Here's how the part is built. I have some questions about the finished solid (model axes, mm). Coordinates: 2 decimals unless noted, no trailing zeros. Write each loop counter-clockwise with the first axis right and the second up, starting at its lowest first coordinate (ties: lowest second). Pieces come first, ordered by that corner, then holes. Notation, with made-up numbers: M 23.5,-13.75 L 55.5,-13.75 A34 cw 55.5,25.25 Z; hole C 14.5,54 d2. An arc over 180 degrees is marked long. Use one line per item in the form item = value. Start each with the question number.
1. I want a section at D-D, the plane z = -30.5. List the corners of the cut face in (x, y) for me.
2. I want a section at C-C, the plane y = -15.5. List the corners of the cut face in (x, z) for me, plus the area to 3 significant figures.
3. I want a section at B-B, the plane x = -67. List the corners of the cut face in (y, z) for me.
4. I'm going to push flat-ended pins straight in: pin 1 Ø12 at (y, z) = (-9.5, -9) entering from +X; pin 2 Ø1 at (x, y) = (28, -15) entering from -Z; pin 3 Ø10 at (y, z) = (-9, -26.5) entering from +X. Where does each tip first touch, or does it pass through?
5. Thinking about a two-plate mould opening in Z: for faces 1 (the face through (47.98, -9.86, 35.17)), 2 (the face through (0, -10, -50)), 3 (the face through (84.87, -9.86, -1.99)), which applies, released by +Z, released by -Z, zero draft, split by the parting line, or undercut?
6. Please list where these lines run through material, in increasing order: line 1 along X through (y, z) = (-7.25, -2); line 2 along X through (y, z) = (-9.5, 12); line 3 along Z through (x, y) = (2, -13.75). Write a range as [from, to].
7. I want a section at A-A, the plane z = 1. List the corners of the cut face in (x, y) for me, plus the area to 3 significant figures.
from build123d import *

# Parameters (mm, degrees)
EXTRUDE_324_DEPTH  = 20
SKETCH1_R          = 15
CUT_EXTRUDE1_DEPTH = 110.201641513


with BuildPart() as part:
    # Эскиз1 → Extrude 324 (new body)
    with BuildSketch(Plane(origin=(0, 0, 0), x_dir=(-1, 0, 0), z_dir=(0, -1, 0))):
        with BuildLine():
            Line((-78.917505692, 23.388614652), (-17.835027079, 46.710938859))
            ThreePointArc((-17.835027079, 46.710938859), (-0.148812417, 49.999778548), (17.556665634, 46.816273793))
            Line((17.556665634, 46.816273793), (78.776887546, 23.857954408))
            ThreePointArc((78.776887546, 23.857954408), (94.998038561, 0.610466623), (79.076996078, -22.84357002))
            Line((79.076996078, -22.84357002), (18.156882698, -46.586775062))
            ThreePointArc((18.156882698, -46.586775062), (0.148812417, -49.999778548), (-17.879254632, -46.694028031))
            Line((-17.879254632, -46.694028031), (-78.939619469, -23.313868793))
            ThreePointArc((-78.939619469, -23.313868793), (-94.99998935, 0.044982802), (-78.917505692, 23.388614652))
        make_face()
    extrude(amount=EXTRUDE_324_DEPTH)

    # Sketch1 → Cut-Extrude1 (cut, through all)
    with BuildSketch(Plane(origin=(0, 0, 0), x_dir=(1, 0, 0), z_dir=(0, 1, 0))):
        with Locations(Location((-69.998554729, 0.449817511, 0), (0, 0, 270))):
            Circle(SKETCH1_R)
        with Locations(Location((69.999992153, 0.033145222, 0), (0, 0, 270))):
            Circle(SKETCH1_R)
    extrude(amount=-CUT_EXTRUDE1_DEPTH, mode=Mode.SUBTRACT)


solid = part.part
Answer list:
q1.outline = M -61.07,-20 L 60.29,-20 L 60.29,0 L -61.07,0 Z
q2.outline = M -79.08,22.84 A25 ccw -78.78,-23.86 L -17.56,-46.82 A50 ccw 17.84,-46.71 L 78.92,-23.39 A25 ccw 78.94,23.31 L 17.88,46.69 A50 ccw -18.16,46.59 Z; hole C -70,-0.45 d30; hole C 70,-0.03 d30
q2.area = 11,700 mm²
q3.outline = M -20,-28.27 L 0,-28.27 L 0,-15.15 L -20,-15.15 Z; M -20,14.25 L 0,14.25 L 0,27.55 L -20,27.55 Z
q4.pin_1 = 94.82
q4.pin_2 = -43.02
q4.pin_3 = 82.81
q5.face_1 = released by +Z
q5.face_2 = released by -Z
q5.face_3 = undercut
q6.line_1 = [-94.95, -84.92], [-55.08, 55.13], [84.87, 94.92]
q6.line_2 = [-91.68, -78.37], [-61.63, 61.04], [78.96, 91.91]
q6.line_3 = [-49.96, 49.96]
q7.outline = M -94.96,-20 L -84.93,-20 L -84.93,0 L -94.96,0 Z; M -55.07,-20 L 55.04,-20 L 55.04,0 L -55.07,0 Z; M 84.96,-20 L 94.98,-20 L 94.98,0 L 84.96,0 Z
q7.area = 2,600 mm²
